Here's how the part is built. I have some questions about the finished solid (model axes, mm). Face numbers are marked on the shaded views. Give positions to 0.01 mm unless a question says otherwise; leave off trailing zeros. Loops run counter-clockwise (first coordinate to the right, second up) from the corner with the lowest first, then second, coordinate; pieces in that order, holes last. Notation, with made-up numbers: (-1.5, -38) - (25.5, -38) arc R8 ccw to (25.5, -28) - close; hole circle Ø4 at (57, 56). An arc over 180 degrees is marked (long way). Put each result on its own line as item: value. Start each with the question number.
from build123d import *

# Parameters (mm, degrees)
BOSS_EXTRUDE1_DEPTH = 22
SKETCH3_R           = 1.75
CUT_EXTRUDE1_DEPTH  = 22
SKETCH4_R           = 3.25
CUT_EXTRUDE2_DEPTH  = 22
FILLET1_R           = 1
SKETCH5_W           = 36.583479506
SKETCH5_H           = 0.5
CUT_EXTRUDE3_DEPTH  = 39


with BuildPart() as part:
    # Sketch2 → Boss-Extrude1 (new body)
    with BuildSketch(Plane(origin=(0, 0, 0), x_dir=(1, 0, 0), z_dir=(0, 1, 0))):
        with BuildLine():
            Line((5, 0), (17.5, 0))
            ThreePointArc((17.5, 0), (0, -17.5), (-17.5, 0))
            Line((-17.5, 0), (-5, 0))
            ThreePointArc((-5, 0), (0, -5), (5, 0))
        make_face()
    extrude(amount=BOSS_EXTRUDE1_DEPTH)

    # Sketch3 → Cut-Extrude1 (cut)
    with BuildSketch(Plane(origin=(0, 0, 0), x_dir=(-1, 0, 0), z_dir=(0, 0, -1))):
        with Locations((11.25, 11)):
            Circle(SKETCH3_R)
        with Locations((-11.25, 11)):
            Circle(SKETCH3_R)
    extrude(amount=-CUT_EXTRUDE1_DEPTH, mode=Mode.SUBTRACT)

    # Sketch4 → Cut-Extrude2 (cut)
    with BuildSketch(Plane(origin=(0, 0, 4.5), x_dir=(-1, 0, 0), z_dir=(0, 0, -1))):
        with Locations((-11.25, 11)):
            Circle(SKETCH4_R)
        with Locations((11.25, 11)):
            Circle(SKETCH4_R)
    extrude(amount=-CUT_EXTRUDE2_DEPTH, mode=Mode.SUBTRACT)

    # Fillet1
    fillet1_edges = [part.edges().sort_by_distance(p)[0] for p in [
        (0, 22, 17.5),
        (0, 0, 17.5),
    ]]
    fillet(fillet1_edges, radius=FILLET1_R)

    # Sketch5 → Cut-Extrude3 (cut)
    with BuildSketch(Plane(origin=(0, 22, 0), x_dir=(1, 0, 0), z_dir=(0, 1, 0))):
        with Locations((-0.146844137, -0.25)):
            Rectangle(SKETCH5_W, SKETCH5_H)
    extrude(amount=-CUT_EXTRUDE3_DEPTH, mode=Mode.SUBTRACT)


solid = part.part
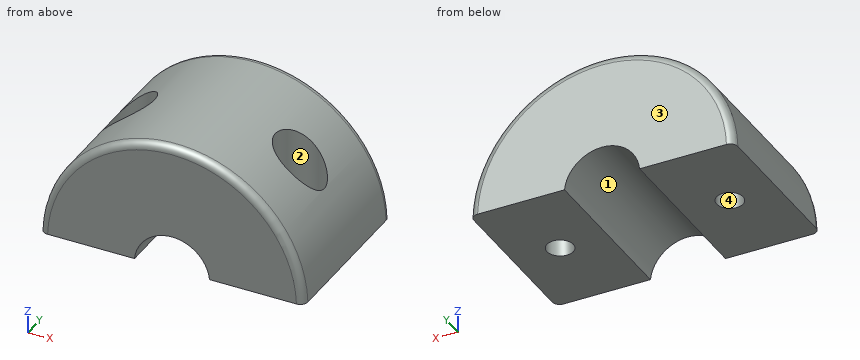
1) Thinking about a two-plate mould opening in Y: for the marked faces 1, 2, 3 and 4, which applies, pulls with the +Y half, pulls with the -Y half, needs draft (parallel to the pull), parting line crosses it, or undercut?
2) Suppose I cut it at A-A on y = 10. Please give me the cut outline in (x, z).
3) I'm going to push flat-ended pins straight in: P1, Ø1.5, axis at x = 2.5, y = 5.5, coming from the -Z side; P2, Ø1.5, axis at y = 4.5, z = 14, coming from the +X side; P3, Ø5, axis at x = -12.5, y = 12, coming from the +Z side. Where does each tip first touch, or does it pass through?
4) Suppose I cut it at C-C on z = 2.75. Give the number of separate pieces and of enclosed holes in the cut face, plus the area to 3 significant figures.
5) I need wall thicknesses on line 1 (Y direction, x = -11.25, z = 2.45); line 2 (Y direction, x = -11.25, z = 11); line 3 (X direction, y = 11, z = 10). Which ranges of each line are inside material? Lowest first, please.
6) Suppose I cut it at B-B on x = 0. Please give me the cut outline in (y, z), plus the area to 3 significant figures.
Ans:
1. face 1: needs draft
1. face 2: undercut
1. face 3: pulls with the +Y half
1. face 4: undercut
2. outline: (-17.49, 0.5) - (-12.69, 0.5) - (-12.69, 4.5) - (-14.34, 4.5) - (-14.34, 10.03) arc R17.5 ccw to start; (-9.81, 0.5) - (-4.97, 0.5) arc R5 cw to (4.97, 0.5) - (9.81, 0.5) - (9.81, 4.5) - (8.16, 4.5) - (8.16, 15.48) arc R17.5 ccw to (-8.16, 15.48) - (-8.16, 4.5) - (-9.81, 4.5) - close; (12.69, 0.5) - (17.49, 0.5) arc R17.5 ccw to (14.34, 10.03) - (14.34, 4.5) - (12.69, 4.5) - close
3. P1: stops at z = 3.8
3. P2: stops at x = 11.43
3. P3: stops at z = 13.27
4. separate pieces: 2
4. enclosed holes: 2
4. area: 557 mm²
5. line 1: y = 0 to 9.25, 12.75 to 22
5. line 2: y = 0 to 7.75, 14.25 to 22
5. line 3: x = -8 to 8
6. outline: (0, 5) - (22, 5) - (22, 16.5) arc R1 ccw to (21, 17.5) - (1, 17.5) arc R1 ccw to (0, 16.5) - close
6. area: 275 mm²
